Could you check a few things on this model? Use its own coordinates, in mm. Face numbers are marked on the shaded views. A direction names the side the tool comes from. Give positions to 0.01 mm unless a question says otherwise; leave off trailing zeros. Loops run counter-clockwise (first coordinate to the right, second up) from the corner with the lowest first, then second, coordinate; pieces in that order, holes last. Notation, with made-up numbers: M 87,50 L 144,50 A11 ccw 144,67 Z; hole C 69.5,87 d8. An arc over 180 degrees is marked long. Return JSON: item names as keys, results as strings. Group by question number.
1. If we mould it in two halves opening along Z, with no side actions, what happens to the marked faces 1, 2 and 3? For each: +Z half, -Z half, draft (parallel to the pull), parting line (faces both ways), or undercut.
2. For the marked faces 4, 5 and 6, which set-ups out of +Z, -Z, +X, -X, +Y, -Y let a thin tool reach every point of the face, with its end or its side?
3. If we section it at C-C (z = 20): Write out the boundary of the cut face in (x, y).
4. For pin 1 (8 mm diameter, centred on x = 27.5, z = 17, fed in from -Y); pin 2 (1.8 mm diameter, centred on x = -1.5, y = 5, fed in from +Z); pin 3 (1.2 mm diameter, centred on y = 1.5, z = 3, fed in from -X); pin 4 (5 mm diameter, centred on y = 8.5, z = 33.5, fed in from -X), each with a flat end and sliding along its axis, tell me the tip position at first contact or that it passes through.
5. If we section it at B-B (x = 34): Write out the boundary of the cut face in (y, z), plus the area to 3 significant figures.
6. Please list where these lines run through material, in increasing order: line 1 (X direction, y = 1.75, z = 17.5); line 2 (Z direction, x = 50.5, y = 3.5); line 3 (X direction, y = 5, z = 23).
7. If we section it at A-A (z = 3.5): Write out the boundary of the cut face in (x, y).
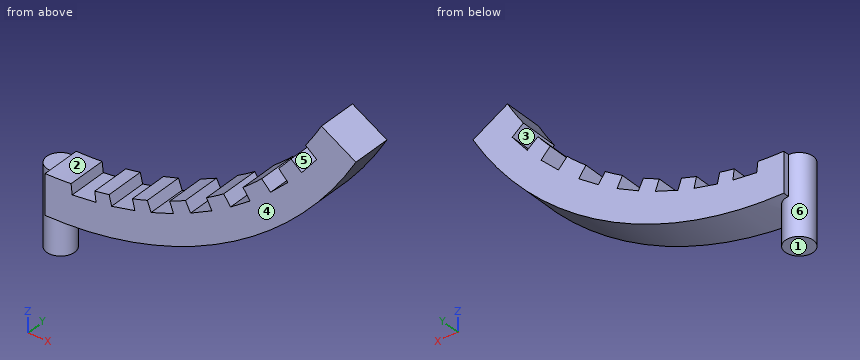
```python
from build123d import *

# Parameters (mm, degrees)
SKETCH001_R                = 3.5
EXTRUDE001_DEPTH           = 10
SKETCH012_W                = 6
SKETCH012_H                = 10
EXTRUDE013_DEPTH           = 2.5
EXTRUDE013_PLACEMENT_ANGLE = 51.18
SKETCH011_W                = 6
SKETCH011_H                = 10
EXTRUDE012_DEPTH           = 2.5
EXTRUDE012_PLACEMENT_ANGLE = 43.68
SKETCH010_W                = 6
SKETCH010_H                = 10
EXTRUDE011_DEPTH           = 2.5
EXTRUDE011_PLACEMENT_ANGLE = 35.16
SKETCH009_W                = 6
SKETCH009_H                = 10
EXTRUDE010_DEPTH           = 2.5
EXTRUDE010_PLACEMENT_ANGLE = 27.42
SKETCH008_W                = 6
SKETCH008_H                = 10
EXTRUDE009_DEPTH           = 2.5
EXTRUDE009_PLACEMENT_ANGLE = 20.22
SKETCH007_W                = 6
SKETCH007_H                = 10
EXTRUDE008_DEPTH           = 2.5
EXTRUDE008_PLACEMENT_ANGLE = 13.32
SKETCH005_W                = 6
SKETCH005_H                = 10
EXTRUDE006_DEPTH           = 2.5
EXTRUDE006_PLACEMENT_ANGLE = 6.6
EXTRUDE002_DEPTH           = 5


with BuildPart() as extrude001:
    # Sketch001 → Extrude001 (new body, symmetric)
    with BuildSketch(Plane.XY):
        Circle(SKETCH001_R)
    extrude(amount=EXTRUDE001_DEPTH, both=True)


with BuildPart() as extrude013:
    # Sketch012 → Extrude013 (new body, symmetric)
    with BuildSketch(Plane.XY):
        Rectangle(SKETCH012_W, SKETCH012_H)
    extrude(amount=EXTRUDE013_DEPTH, both=True)


with BuildPart() as extrude013_1:
    # Extrude013 placement: moved
    add(extrude013.part.moved(Location((64.277333, 0, 40.782745))).rotate(Axis((64.277333, 0, 40.782745), (0, -1, 0)), EXTRUDE013_PLACEMENT_ANGLE))


with BuildPart() as extrude012:
    # Sketch011 → Extrude012 (new body, symmetric)
    with BuildSketch(Plane.XY):
        Rectangle(SKETCH011_W, SKETCH011_H)
    extrude(amount=EXTRUDE012_DEPTH, both=True)


with BuildPart() as extrude012_1:
    # Extrude012 placement: moved
    add(extrude012.part.moved(Location((56.976975, 0, 32.835318))).rotate(Axis((56.976975, 0, 32.835318), (0, -1, 0)), EXTRUDE012_PLACEMENT_ANGLE))


with BuildPart() as extrude011:
    # Sketch010 → Extrude011 (new body, symmetric)
    with BuildSketch(Plane.XY):
        Rectangle(SKETCH010_W, SKETCH010_H)
    extrude(amount=EXTRUDE011_DEPTH, both=True)


with BuildPart() as extrude011_1:
    # Extrude011 placement: moved
    add(extrude011.part.moved(Location((47.50859, 0, 25.052362))).rotate(Axis((47.50859, 0, 25.052362), (0, -1, 0)), EXTRUDE011_PLACEMENT_ANGLE))


with BuildPart() as extrude010:
    # Sketch009 → Extrude010 (new body, symmetric)
    with BuildSketch(Plane.XY):
        Rectangle(SKETCH009_W, SKETCH009_H)
    extrude(amount=EXTRUDE010_DEPTH, both=True)


with BuildPart() as extrude010_1:
    # Extrude010 placement: moved
    add(extrude010.part.moved(Location((37.992047, 0, 19.268488))).rotate(Axis((37.992047, 0, 19.268488), (0, -1, 0)), EXTRUDE010_PLACEMENT_ANGLE))


with BuildPart() as extrude009:
    # Sketch008 → Extrude009 (new body, symmetric)
    with BuildSketch(Plane.XY):
        Rectangle(SKETCH008_W, SKETCH008_H)
    extrude(amount=EXTRUDE009_DEPTH, both=True)


with BuildPart() as extrude009_1:
    # Extrude009 placement: moved
    add(extrude009.part.moved(Location((28.514126, 0, 15.084274))).rotate(Axis((28.514126, 0, 15.084274), (0, -1, 0)), EXTRUDE009_PLACEMENT_ANGLE))


with BuildPart() as extrude008:
    # Sketch007 → Extrude008 (new body, symmetric)
    with BuildSketch(Plane.XY):
        Rectangle(SKETCH007_W, SKETCH007_H)
    extrude(amount=EXTRUDE008_DEPTH, both=True)


with BuildPart() as extrude008_1:
    # Extrude008 placement: moved
    add(extrude008.part.moved(Location((19.007128, 0, 12.219373))).rotate(Axis((19.007128, 0, 12.219373), (0, -1, 0)), EXTRUDE008_PLACEMENT_ANGLE))


with BuildPart() as extrude006:
    # Sketch005 → Extrude006 (new body, symmetric)
    with BuildSketch(Plane.XY):
        Rectangle(SKETCH005_W, SKETCH005_H)
    extrude(amount=EXTRUDE006_DEPTH, both=True)


with BuildPart() as extrude006_1:
    # Extrude006 placement: moved
    add(extrude006.part.moved(Location((9.482315, 0, 10.546747))).rotate(Axis((9.482315, 0, 10.546747), (0, -1, 0)), EXTRUDE006_PLACEMENT_ANGLE))


with BuildPart() as fusion:
    # Sketch002 → Extrude002 (new body, symmetric)
    with BuildSketch(Plane.XZ):
        with BuildLine():
            ThreePointArc((0, 0), (45.00001, 12.057678), (77.942322, 44.999938))
            Line((69.282072, 49.999945), (77.942322, 44.999938))
            ThreePointArc((0, 10), (40.000013, 20.717934), (69.282072, 49.999945))
            Line((0, 10), (0, 0))
        make_face()
    extrude(amount=EXTRUDE002_DEPTH, both=True)

    # Cut: cut Extrude006
    add(extrude006_1.part, mode=Mode.SUBTRACT)

    # Cut001: cut Extrude008
    add(extrude008_1.part, mode=Mode.SUBTRACT)

    # Cut002: cut Extrude009
    add(extrude009_1.part, mode=Mode.SUBTRACT)

    # Cut003: cut Extrude010
    add(extrude010_1.part, mode=Mode.SUBTRACT)

    # Cut004: cut Extrude011
    add(extrude011_1.part, mode=Mode.SUBTRACT)

    # Cut005: cut Extrude012
    add(extrude012_1.part, mode=Mode.SUBTRACT)

    # Cut006: cut Extrude013
    add(extrude013_1.part, mode=Mode.SUBTRACT)

    # Fusion: union Extrude001
    add(extrude001.part)


with BuildPart() as fusion_1:
    # Fusion placement: moved
    add(fusion.part.moved(Location((0, 6, 0))))


solid = fusion_1.part
```
Answer:
{
 "1": {"face 1": "-Z half", "face 2": "+Z half", "face 3": "undercut"},
 "2": {"face 4": "+Z, -Z, +X, -X, -Y", "face 5": "+Z, +Y, -Y", "face 6": "-Z"},
 "3": {"outline": "M 40.99,1 L 56.57,1 L 56.57,11 L 40.99,11 Z"},
 "4": {"pin 1": "stops at y = 1", "pin 2": "stops at z = 10", "pin 3": "stops at x = 0", "pin 4": "stops at x = 54.03"},
 "5": {"outline": "M 1,6.67 L 11,6.67 L 11,17.58 L 1,17.58 Z", "area": "109 mm²"},
 "6": {"line 1": "x = 33.82 to 35.53, 40.01 to 53.33", "line 2": "z = 15.5 to 24.1, 26.02 to 27.95", "line 3": "x = 43.72 to 45.28, 48.94 to 60.09"},
 "7": {"outline": "M 0,1 L 24.85,1 L 24.85,11 L 0,11 L 0,9.5 A3.5 ccw 0,2.5 Z"}
}
